from build123d import *

# Parameters (mm, degrees)
BOX184_W               = 6
BOX184_H               = 6.45
BOX184_DEPTH           = 1.05
BOX183_W               = 6
BOX183_H               = 6.5
BOX183_DEPTH           = 1.15
CUT092_PLACEMENT_ANGLE = 148


with BuildPart() as small_cu_gnd_electrode076:
    # Box184 → Box184 (new body)
    with BuildSketch(Plane.XY.offset(0.05)):
        with Locations((3, 3.225)):
            Rectangle(BOX184_W, BOX184_H)
    extrude(amount=BOX184_DEPTH)


with BuildPart() as small_cu_electrode_short_axis_gnd009:
    # Box183 → Box183 (new body)
    with BuildSketch(Plane.XY):
        with Locations((3, 3.25)):
            Rectangle(BOX183_W, BOX183_H)
    extrude(amount=BOX183_DEPTH)

    # Cut092: cut Small Cu GND Electrode076
    add(small_cu_gnd_electrode076.part, mode=Mode.SUBTRACT)


with BuildPart() as small_cu_electrode_short_axis_gnd009_1:
    # Cut092 placement: moved
    add(small_cu_electrode_short_axis_gnd009.part.moved(Location((13.251142, 19.640047, 1.59))).rotate(Axis((13.251142, 19.640047, 1.59), (0, 0, 1)), CUT092_PLACEMENT_ANGLE))


solid = small_cu_electrode_short_axis_gnd009_1.part
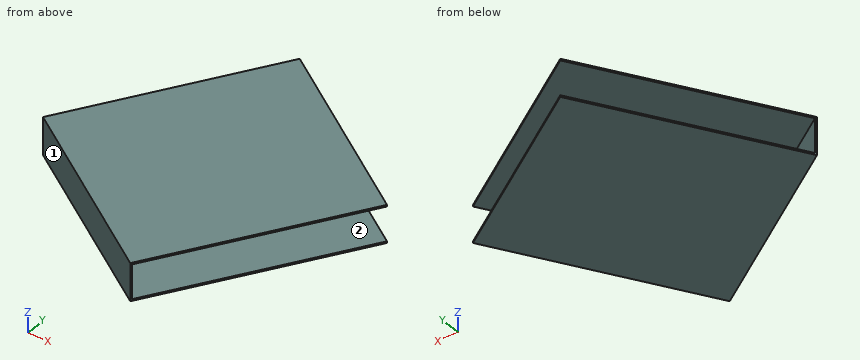
Build history of the part. All positions in model axes, mm. Face numbers are marked on the shaded views. A direction names the side the tool comes from. Coordinates: 2 decimals unless noted, no trailing zeros. Order: outer loops, then holes, each group sorted by start corner. A loop starts at its lowest first (then second) coordinate and runs counter-clockwise, first axis right, second up. Notation, with made-up numbers: (79.25, -14.75) - (125.25, -14.75) arc R14 ccw to (125.25, 1.25) - close; hole circle Ø3 at (43.5, 23.25). An arc over 180 degrees is marked (long way). Write item = value, one per line. Start each with the question number.
1) Saw through at C-C on z = 2.55. Write the cut outline in (x, y).
2) 3-axis set-ups, long thin cutter, end or side, ignore diameter. For the marked faces 1 and 2: which of +Z, -Z, +X, -X, +Y, -Y reach the whole face in a straight line?
3) Saw through at B-B on y = 20. Write the cut outline in (x, z).
4) Saw through at D-D on y = 16. Write the cut outline in (x, z), then the cut area to 3 significant figures.
5) Saw through at A-A on x = 10.25. Write the cut outline in (y, z), then the cut area to 3 significant figures.
From the geometry:
q1.outline = (4.72, 17.31) - (9.81, 14.13) - (9.83, 14.17) - (4.74, 17.35) - close
q2.face_1 = +Z, -Z, -X, -Y
q2.face_2 = +X, +Y
q3.outline = (6.4, 1.59) - (12.68, 1.59) - (12.68, 1.64) - (6.4, 1.64) - close; (6.4, 2.69) - (12.68, 2.69) - (12.68, 2.74) - (6.4, 2.74) - close
q4.outline = (6.81, 1.59) - (10.98, 1.59) - (10.98, 1.64) - (6.9, 1.64) - (6.9, 2.69) - (10.98, 2.69) - (10.98, 2.74) - (6.81, 2.74) - close
q4.area = 0.516 mm^2
q5.outline = (14.84, 1.59) - (21.52, 1.59) - (21.52, 1.64) - (14.84, 1.64) - close; (14.84, 2.69) - (21.52, 2.69) - (21.52, 2.74) - (14.84, 2.74) - close
q5.area = 0.668 mm^2
